from build123d import *

# Parameters (mm, degrees)
SKETCH2_R           = 0.95
SKETCH2_R_2         = 0.7
BOSS_EXTRUDE1_DEPTH = 4
SKETCH3_W           = 16.2
SKETCH3_H           = 9.945
CUT_EXTRUDE2_DEPTH  = 2


with BuildPart() as part:
    # Sketch2 → Boss-Extrude1 (new body)
    with BuildSketch(Plane.XY):
        with BuildLine():
            Line((0, 9.945), (0, 6))
            Line((0, 6), (4, 6))
            Line((4, 6), (4, 4))
            Line((4, 4), (0, 4))
            Line((0, 4), (0, 2))
            ThreePointArc((0, 2), (0.585786438, 0.585786438), (2, 0))
            Line((2, 0), (14.2, 0))
            ThreePointArc((14.2, 0), (15.614213562, 0.585786438), (16.2, 2))
            Line((16.2, 2), (16.2, 4))
            Line((16.2, 4), (12.2, 4))
            Line((12.2, 4), (12.2, 6))
            Line((12.2, 6), (16.2, 6))
            Line((16.2, 6), (16.2, 9.945))
            ThreePointArc((16.2, 9.945), (14.735533906, 13.480533906), (11.2, 14.945))
            Line((11.2, 14.945), (5, 14.945))
            ThreePointArc((5, 14.945), (1.464466094, 13.480533906), (0, 9.945))
        make_face()
        with Locations((13.25, 8)):
            Circle(SKETCH2_R, mode=Mode.SUBTRACT)
        with Locations((13.25, 2)):
            Circle(SKETCH2_R, mode=Mode.SUBTRACT)
        with Locations((13.2, 11.942)):
            Circle(SKETCH2_R_2, mode=Mode.SUBTRACT)
        with Locations((3, 11.942)):
            Circle(SKETCH2_R_2, mode=Mode.SUBTRACT)
        with Locations((2.95, 2)):
            Circle(SKETCH2_R, mode=Mode.SUBTRACT)
        with Locations((2.95, 8)):
            Circle(SKETCH2_R, mode=Mode.SUBTRACT)
    extrude(amount=BOSS_EXTRUDE1_DEPTH)

    # Sketch3 → Cut-Extrude2 (cut)
    with BuildSketch(Plane(origin=(0, 0, 4), x_dir=(-1, 0, 0), z_dir=(0, 0, -1))):
        with Locations((-8.1, 4.9725)):
            Rectangle(SKETCH3_W, SKETCH3_H)
    extrude(amount=CUT_EXTRUDE2_DEPTH, mode=Mode.SUBTRACT)


solid = part.part
The model under review builds one solid part; all positions refer to its coordinate system, in mm. A direction names the side the tool comes from. Round coordinates to 2 decimals unless told otherwise and drop trailing zeros. Order: outer loops, then holes, each group sorted by start corner. A loop starts at its lowest first (then second) coordinate and runs counter-clockwise, first axis right, second up. Notation, with made-up numbers: (-10, 74.5) -> (4, 74.5) arc R19 ccw to (4, 108.5) -> close; hole circle Ø5 at (-24, 43.25). An arc over 180 degrees is marked (long way). Use CSV: the item, a comma, the result in double quotes. Start each with the question number.
(1) Consider section D-D on z = 0.35. Write out the cut boundary in (x, y) (3 decimals), and give its area (3 significant figures).
(2) Consider section B-B on x = 13.25. Write out the cut boundary in (y, z) (3 decimals), and give its area (3 significant figures).
(3) Mouldability with a two-part tool opening along X and no side actions: class faces 6 (the face through (8, 8, 0)), 7 (the face through (14.156, 2.285, 0.986)), 8 (the face through (14.156, 8.285, 0.986)), 9 (the face through (0.57, 0.6, 0.99)) as pulls with the +X half, pulls with the -X half, needs draft (parallel to the pull), parting line crosses it, or undercut.
(4) Consider section C-C on x = 10. Write out the cut boundary in (y, z) (3 decimals), and give its area (3 significant figures).
(5) Tool access review of faces 1 (the face through (14, 6, 1)), 2 (the face through (2, 4, 1)), 3 (the face through (16.2, 8, 1)), 4 (the face through (3.856, 2.285, 0.986)), 5 (the face through (8, 9.945, 3)): name each direction out of +Z, -Z, +X, -X, +Y, -Y from which nothing blocks a thin tool from reaching the whole face with its end or side.
(6) Wall thickness on probe 1 along X at (y, z) = (2, 0.75); probe 2 along Y at (x, z) = (13.25, 1.35); probe 3 along X at (y, z) = (11.75, 0.6): over which ranges is each line inside the solid? List them lowest first. Write a range as from..to.
(7) Insertion check: pin 1 (1.6 mm diameter, centred on x = 14.5, z = 1, fed in from -Y); pin 2 (0.6 mm diameter, centred on x = 2.5, z = 0.5, fed in from +Y) (3 decimals); pin 3 (2.5 mm diameter, centred on x = 2.95, y = 2, fed in from +Z); pin 4 (0.6 mm diameter, centred on x = 14, z = 0.5, fed in from +Y). Each pin has a flat end and moves straight along its axis. Give the tip position at first contact, or say it passes through.
(8) Consider section A-A on y = 8. Write out the cut boundary in (x, z), and give its area (3 significant figures).
Responses:
1,outline,"(0, 2) arc R2 ccw to (2, 0) -> (14.2, 0) arc R2 ccw to (16.2, 2) -> (16.2, 4) -> (12.2, 4) -> (12.2, 6) -> (16.2, 6) -> (16.2, 9.945) arc R5 ccw to (11.2, 14.945) -> (5, 14.945) arc R5 ccw to (0, 9.945) -> (0, 6) -> (4, 6) -> (4, 4) -> (0, 4) -> close; hole circle Ø1.9 at (2.95, 2); hole circle Ø1.9 at (2.95, 8); hole circle Ø1.4 at (3, 11.942); hole circle Ø1.9 at (13.25, 2); hole circle Ø1.9 at (13.25, 8); hole circle Ø1.4 at (13.2, 11.942)"
1,area,"199 mm²"
2,outline,"(0, 0) -> (1.05, 0) -> (1.05, 2) -> (0, 2) -> close; (2.95, 0) -> (4, 0) -> (4, 2) -> (2.95, 2) -> close; (6, 0) -> (7.05, 0) -> (7.05, 2) -> (6, 2) -> close; (8.95, 0) -> (11.244, 0) -> (11.244, 4) -> (9.945, 4) -> (9.945, 2) -> (8.95, 2) -> close; (12.64, 0) -> (14.505, 0) -> (14.505, 4) -> (12.64, 4) -> close"
2,area,"20.9 mm²"
3,face 6,"needs draft"
3,face 7,"undercut"
3,face 8,"undercut"
3,face 9,"pulls with the -X half"
4,outline,"(0, 0) -> (14.945, 0) -> (14.945, 4) -> (9.945, 4) -> (9.945, 2) -> (0, 2) -> close"
4,area,"39.9 mm²"
5,face 1,"+Z, -Z, +X"
5,face 2,"+Z, -Z, -X"
5,face 3,"+Z, -Z, +X, +Y, -Y"
5,face 4,"+Z, -Z"
5,face 5,"+Z, +X, -X, -Y"
6,probe 1,"0..2, 3.9..12.3, 14.2..16.2"
6,probe 2,"0..1.05, 2.95..4, 6..7.05, 8.95..11.24, 12.64..14.51"
6,probe 3,"0.34..2.33, 3.67..12.53, 13.87..15.86"
7,pin 1,"y = 0"
7,pin 2,"y = 14.435"
7,pin 3,"z = 2"
7,pin 4,"y = 14.28"
8,outline,"(0, 0) -> (2, 0) -> (2, 2) -> (0, 2) -> close; (3.9, 0) -> (12.3, 0) -> (12.3, 2) -> (3.9, 2) -> close; (14.2, 0) -> (16.2, 0) -> (16.2, 2) -> (14.2, 2) -> close"
8,area,"24.8 mm²"
